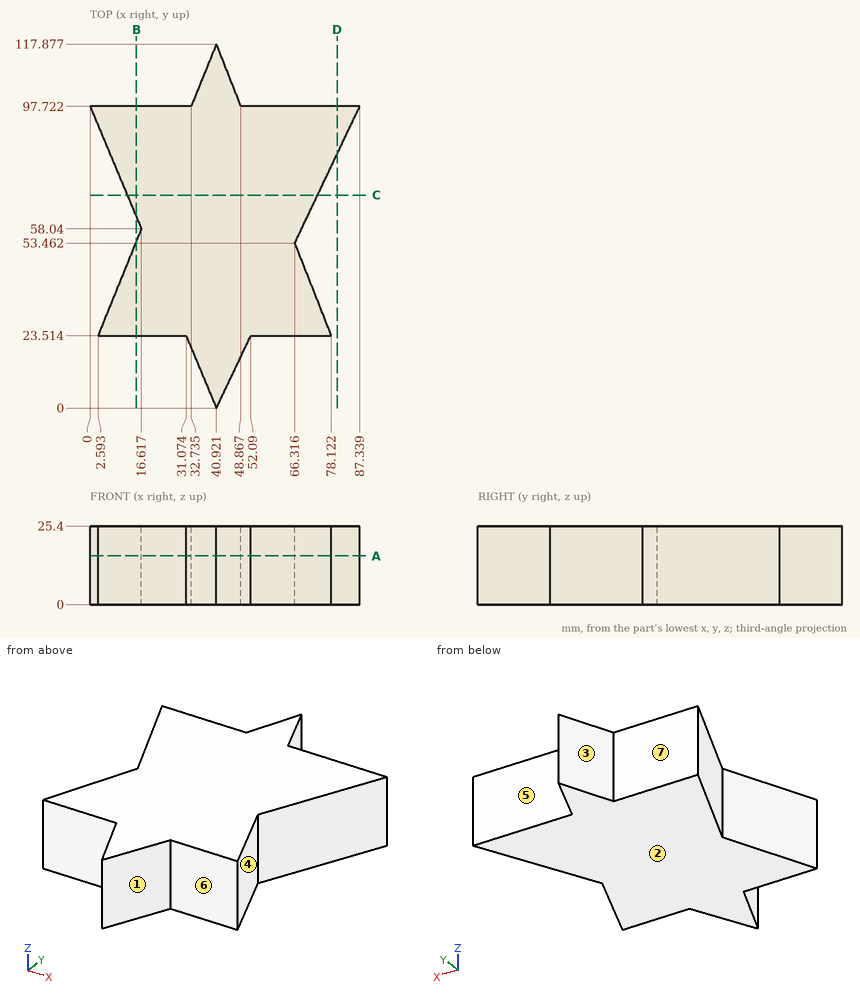
Check sheet for the drawn part. Datum: minimum x, y, z corner. Units: mm. A direction names the side the tool comes from. Coordinates: 2 decimals unless noted, no trailing zeros. Order: outer loops, then holes, each group sorted by start corner. A loop starts at its lowest first (then second) coordinate and runs counter-clockwise, first axis right, second up. Notation, with made-up numbers: (9, 59) - (31, 59) arc R16 ccw to (31, 90) - close; hole circle Ø9 at (-37.5, 35.25). An arc over 180 degrees is marked (long way). Return JSON: item names as keys, results as strings.
(1) Section check C-C, the plane y = 69. Record the cut outline in (x, z), and give its area (3 significant figures).
Filled sheet:
{"outline": "(12.03, 0) - (73.7, 0) - (73.7, 25.4) - (12.03, 25.4) - close", "area": "1,570 mm^2"}
(2) Section check A-A, the plane z = 15.75. Record the cut outline in (x, y) (1 decimal), and give its area (3 significant figures).
Filled sheet:
{"outline": "(0, 97.7) - (16.6, 58) - (2.6, 23.5) - (31.1, 23.5) - (40.9, 0) - (52.1, 23.5) - (78.1, 23.5) - (66.3, 53.5) - (87.3, 97.7) - (48.9, 97.7) - (40.9, 117.9) - (32.7, 97.7) - close", "area": "5,310 mm^2"}
(3) Thickness scan on line 1 along Y through (x, z) = (23, 18.75) (1 decimal); line 2 along Y through (x, z) = (15.5, 1) (1 decimal); line 3 along X through (y, z) = (39, 6). Record the ranges inside material, lowest first.
Filled sheet:
{"line 1": "y = 23.5 to 97.7", "line 2": "y = 23.5 to 55.3, 60.7 to 97.7", "line 3": "x = 8.88 to 72.02"}
(4) Go/stop test with flat-tipped pins: pin 1 (12 mm diameter, centred on y = 103, z = 3, fed in from -X); pin 2 (3 mm diameter, centred on x = 35, z = 19, fed in from -Y) (1 decimal); pin 3 (12.5 mm diameter, centred on x = 66, z = 8.5, fed in from -Y). Record where each tip stops, or that it passes through.
Filled sheet:
{"pin 1": "stops at x = 0", "pin 2": "stops at y = 10.6", "pin 3": "stops at y = 23.51"}
(5) Mould release check, pull along Y, two halves, no side actions. Record for the marked faces 1, 2, 3 and 4: pulls with the +Y half, pulls with the -Y half, needs draft (parallel to the pull), parting line crosses it, or undercut.
Filled sheet:
{"face 1": "pulls with the -Y half", "face 2": "needs draft", "face 3": "pulls with the +Y half", "face 4": "undercut"}
(6) Section check B-B, the plane x = 15. Record the cut outline in (y, z) (1 decimal).
Filled sheet:
{"outline": "(23.5, 0) - (54.1, 0) - (54.1, 25.4) - (23.5, 25.4) - close; (61.9, 0) - (97.7, 0) - (97.7, 25.4) - (61.9, 25.4) - close"}
(7) Access from +Z, -Z, +X, -X, +Y, -Y to the whole of each face (thin tool, end or side, straight path). Record for the marked faces 5, 6 and 7.
Filled sheet:
{"face 5": "+Z, -Z, +X, +Y", "face 6": "+Z, -Z, +X, -Y", "face 7": "+Z, -Z, -X, +Y"}
(8) Section check D-D, the plane x = 80. Record the cut outline in (y, z).
Filled sheet:
{"outline": "(82.27, 0) - (97.72, 0) - (97.72, 25.4) - (82.27, 25.4) - close"}
